```python
from build123d import *

# Parameters (mm, degrees)
SKETCH_1_W          = 58.5
SKETCH_1_H          = 28
EXTRUDE_1_DEPTH     = 1.5
SKETCH_2_R          = 1
CUT_EXTRUDE_1_DEPTH = 1.5
EXTRUDE_2_DEPTH     = 25
SKETCH_4_W          = 16
SKETCH_4_H          = 3
EXTRUDE_3_DEPTH     = 11
SKETCH_5_W          = 8
SKETCH_5_H          = 7.5
SKETCH_5_W_2        = 9
EXTRUDE_4_DEPTH     = 4


with BuildPart() as part:
    # Эскиз1 → Бобышка-Вытянуть1 (new body)
    with BuildSketch(Plane(origin=(0, 0, 0), x_dir=(1, 0, 0), z_dir=(0, 1, 0))):
        with Locations((-29.25, 14)):
            Rectangle(SKETCH_1_W, SKETCH_1_H)
    extrude(amount=EXTRUDE_1_DEPTH)

    # Эскиз2 → Вырез-Вытянуть1 (cut)
    with BuildSketch(Plane(origin=(0, 1.5, 0), x_dir=(1, 0, 0), z_dir=(0, 1, 0))):
        with Locations(Location((-3, 12.5, 0), (0, 0, 270))):
            Circle(SKETCH_2_R)
        with Locations(Location((-41.5, 25.5, 0), (0, 0, 270))):
            Circle(SKETCH_2_R)
    extrude(amount=-CUT_EXTRUDE_1_DEPTH, mode=Mode.SUBTRACT)

    # Эскиз3 → Бобышка-Вытянуть2 (add)
    with BuildSketch(Plane(origin=(0, 1.5, 0), x_dir=(1, 0, 0), z_dir=(0, 1, 0))):
        Polygon((0, 0), (0, 8), (-50.5, 8), (-50.5, 28), (-58.5, 28), (-58.5, 0), align=None)
    extrude(amount=EXTRUDE_2_DEPTH)

    # Эскиз4 → Бобышка-Вытянуть3 (add)
    with BuildSketch(Plane(origin=(0, 1.5, 0), x_dir=(1, 0, 0), z_dir=(0, 1, 0))):
        with Locations((-19, 26.5)):
            Rectangle(SKETCH_4_W, SKETCH_4_H)
    extrude(amount=EXTRUDE_3_DEPTH)

    # Эскиз5 → Бобышка-Вытянуть4 (add)
    with BuildSketch(Plane(origin=(0, 1.5, 0), x_dir=(1, 0, 0), z_dir=(0, 1, 0))):
        with Locations((4, 21.75)):
            Rectangle(SKETCH_5_W, SKETCH_5_H)
        with Locations((-4.5, 21.75)):
            Rectangle(SKETCH_5_W_2, SKETCH_5_H)
    extrude(amount=EXTRUDE_4_DEPTH)


solid = part.part
```
Can you work these out from the model? Positions are in its coordinate system, mm. A direction names the side the tool comes from. Coordinates: 2 decimals unless noted, no trailing zeros. Loops run counter-clockwise (first coordinate to the right, second up) from the corner with the lowest first, then second, coordinate; pieces in that order, holes last.
Item 1: Suppose I cut it at A-A (z = -12.5). Please give me the cut outline in (x, y), then the cut area to 3 significant figures.
Answers below:
outline: (-58.5, 0) - (-4, 0) - (-4, 1.5) - (-50.5, 1.5) - (-50.5, 26.5) - (-58.5, 26.5) - close; (-2, 0) - (0, 0) - (0, 1.5) - (-2, 1.5) - close
area: 285 mm2
Item 2: Which directions (+Z, -Z, +X, -X, +Y, -Y) give clear straight access to the entire face, cutting with the end or side of a thin tool? Please do faces 4 (the face through (-36, 26.5, -5)), 5 (the face through (-25, 14, -8)), 6 (the face through (4, 1.5, -22)), 7 (the face through (-9, 3, -22)), 8 (the face through (-1, 5.5, -22)).
Answers below:
face 4: +Z, -Z, +X, -X, +Y
face 5: +X, +Y
face 6: +Z, -Z, +X, -Y
face 7: -Z, +Y
face 8: -Z, +X, +Y
Item 3: Suppose I cut it at D-D (y = 15.5). Please give me the cut outline in (x, z), then the cut area to 3 significant figures.
Answers below:
outline: (-58.5, -28) - (-50.5, -28) - (-50.5, -8) - (0, -8) - (0, 0) - (-58.5, 0) - close
area: 628 mm2
Item 4: Suppose I cut it at C-C (x = -5.5). Please give me the cut outline in (y, z), then the cut area to 3 significant figures.
Answers below:
outline: (0, -28) - (1.5, -28) - (1.5, -25.5) - (5.5, -25.5) - (5.5, -18) - (1.5, -18) - (1.5, -8) - (26.5, -8) - (26.5, 0) - (0, 0) - close
area: 272 mm2
Item 5: If we mould it in two halves opening along Z, with no side actions, what happens to faces 1 (the face through (0, 3, -25.5)), 2 (the face through (-26, 1.5, -18)), 3 (the face through (-30, 0, -14))? For each: released by +Z, released by -Z, zero draft, split by the parting line, or undercut.
Answers below:
face 1: released by -Z
face 2: undercut
face 3: zero draft
Item 6: Suppose I cut it at B-B (x = -41.5). Please give me the cut outline in (y, z).
Answers below:
outline: (0, -28) - (1.5, -28) - (1.5, -26.5) - (0, -26.5) - close; (0, -24.5) - (1.5, -24.5) - (1.5, -8) - (26.5, -8) - (26.5, 0) - (0, 0) - close
Item 7: I'm going to push flat-ended pins straight in: pin 1 (6 mm diameter, centred on y = 11.5, z = -14, fed in from +X); pin 2 (1.5 mm diameter, centred on x = -34, y = 22.5, fed in from -Z); pin 3 (6 mm diameter, centred on x = -34, z = -19.5, fed in from +Y). Where does each tip first touch, or does it pass through?
Answers below:
pin 1: stops at x = -50.5
pin 2: stops at z = -8
pin 3: stops at y = 1.5
Item 8: Please list where these lines run through material, in increasing order: L1, parallel to X at y = 0.3, z = -12.5; L2, parallel to Z at x = -29, y = 14.75; L3, parallel to Y at x = -18, z = -9.25.
Answers below:
L1: x = -58.5 to -4, -2 to 0
L2: z = -8 to 0
L3: y = 0 to 1.5
